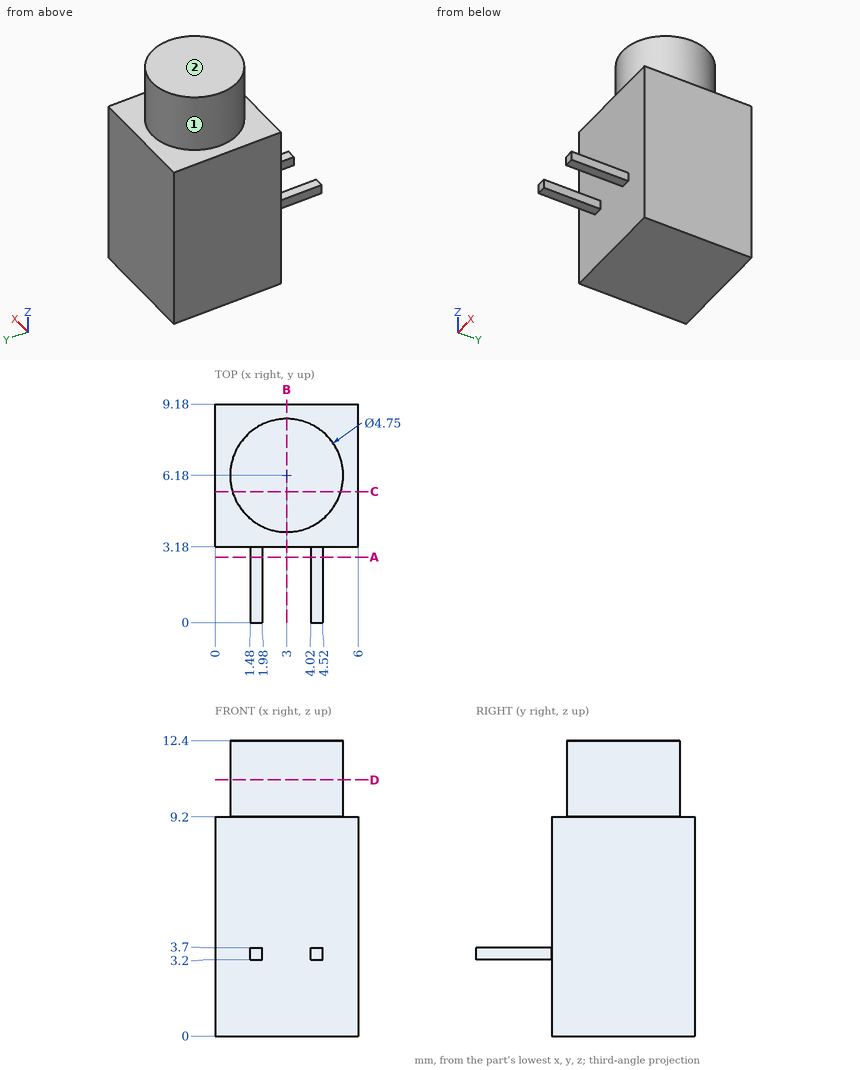
Check sheet for the drawn part. Datum: minimum x, y, z corner. Units: mm. A direction names the side the tool comes from. Give positions to 0.01 mm unless a question says otherwise; leave off trailing zeros. Write each loop counter-clockwise with the first axis right and the second up, starting at its lowest first coordinate (ties: lowest second). Pieces come first, ordered by that corner, then holes. Notation, with made-up numbers: M 27.5,47 L 63.5,47 A21 ccw 63.5,84 Z; hole C -28.5,-6.5 d8. An arc over 180 degrees is marked long. One line per question, with ' | ' between items.
1) Section check B-B on x = 3. Enter the section's corners in (y, z) (3 decimals), plus the area to 3 significant figures.
Result:
outline: M 3.18,0 L 9.18,0 L 9.18,9.2 L 8.555,9.2 L 8.555,12.4 L 3.805,12.4 L 3.805,9.2 L 3.18,9.2 Z | area: 70.4 mm2
2) Section check D-D on z = 10.75. Enter the section's corners in (x, y) (3 decimals).
Result:
outline: C 3,6.18 d4.75
3) Gauge pin test, flat ends, axial feed: pin 1 Ø0.6 at (y, z) = (2.5, 3.5) entering from +X; pin 2 Ø1.5 at (x, z) = (0.5, 4.5) entering from -Y; pin 3 Ø0.6 at (y, z) = (1, 3.5) entering from -X; pin 4 Ø1 at (x, y) = (5.5, 5.5) entering from -Z. Record the tip position at first contact, or that the pin passes through.
Result:
pin 1: stops at x = 4.52 | pin 2: stops at y = 3.18 | pin 3: stops at x = 1.48 | pin 4: stops at z = 0
4) Set-up check for the marked faces 1 and 2: record each of +Z, -Z, +X, -X, +Y, -Y from which the full face is reachable in a straight line by a thin tool's end or side.
Result:
face 1: +Z | face 2: +Z, +X, -X, +Y, -Y
5) Section check A-A on y = 2.75. Enter the section's corners in (x, z).
Result:
outline: M 1.48,3.2 L 1.98,3.2 L 1.98,3.7 L 1.48,3.7 Z; M 4.02,3.2 L 4.52,3.2 L 4.52,3.7 L 4.02,3.7 Z
6) Thickness scan on line 1 along Z through (x, y) = (3.55, 8.75); line 2 along Y through (x, z) = (4.75, 5); line 3 along X through (y, z) = (8, 11.25). Record the ranges inside material, lowest first. Write a range as [from, to].
Result:
line 1: z = [0, 9.2] | line 2: y = [3.18, 9.18] | line 3: x = [1.47, 4.53]
7) Section check C-C on y = 5.5. Enter the section's corners in (x, z).
Result:
outline: M 0,0 L 6,0 L 6,9.2 L 5.28,9.2 L 5.28,12.4 L 0.72,12.4 L 0.72,9.2 L 0,9.2 Z
